The listing builds one solid part. Answer for the finished solid, in the listing's coordinates (mm). Coordinates: 2 decimals unless noted, no trailing zeros. Loops run counter-clockwise (first coordinate to the right, second up) from the corner with the lowest first, then second, coordinate; pieces in that order, holes last. Notation, with made-up numbers: M 10,23 L 15,23 A26 ccw 15,49 Z; hole C 76.5,32 d4. An arc over 180 degrees is marked long. Answer as a JSON object with one key per item and string values. Group by question number.
1. A cutting plane is placed at B-B on x = 2. Give the vertices of the cut face in (y, z).
2. Given pin 1 (6 mm diameter, centred on x = -53.5, y = -24, fed in from +Z); pin 2 (3 mm diameter, centred on x = 16.5, z = 48.5, fed in from +Y); pin 3 (8 mm diameter, centred on y = 22, z = 85.5, fed in from +X); pin 4 (12 mm diameter, centred on x = 22, y = -32.5, fed in from +Z), each flat-ended and moving along its own axis, determine where each tip first touches the part or whether it passes through.
3. A cutting plane is placed at A-A on y = 0. Give the vertices of the cut face in (x, z).
4. A cutting plane is placed at C-C on z = 98.5. Give the vertices of the cut face in (x, y).
5. A cutting plane is placed at D-D on y = 29.5. Give the vertices of the cut face in (x, z).
6. Straight lines are drawn through the part: L1, parallel to Z at x = -23.5, y = -27; L2, parallel to X at y = -11.5, z = 15.5; L3, parallel to Y at x = -52.5, z = 46.5. For each, find the intervals that lie inside material, in ascending order.
from build123d import *

# Parameters (mm, degrees)
F2_T          = -1.2
F3_R          = 17
F4_DEPTH      = 25
F4_DEPTH_BACK = 25


with BuildPart() as f1:
    # F0 (on Front) → F1 (revolve)
    with BuildSketch(Plane.XZ):
        with BuildLine():
            Line((-16.5, 0), (0, 0))
            Line((0, 0), (0, 127))
            Line((0, 127), (-35, 127))
            ThreePointArc((-35, 127), (-68.5223503683, 57.269382033), (-16.5, 0))
        make_face()
    revolve(axis=Axis((0, 0, 63.5), (0, 0, 1)))

    # F2
    f2_openings = [f1.faces().sort_by_distance(p)[0] for p in [
        (0, 0, 127),
    ]]
    offset(amount=F2_T, openings=f2_openings)

    # F3 (on face) → F4 (cut, two sides)
    with BuildSketch(Plane.XY.offset(1.2)) as f4_sk:
        Circle(F3_R)
    extrude(amount=-F4_DEPTH, mode=Mode.SUBTRACT)
    extrude(f4_sk.sketch, amount=F4_DEPTH_BACK, mode=Mode.SUBTRACT)


solid = f1.part
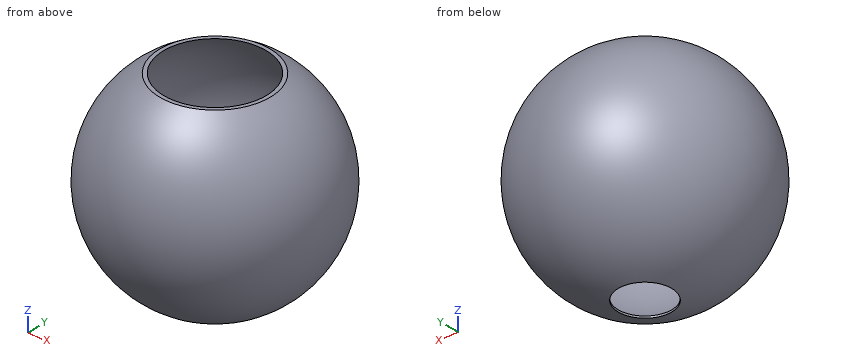
From the geometry:
{
 "1": {"outline": "M -34.94,127 A69.22 ccw -16.88,0.12 L -16.88,1.36 A68.02 cw -32.5,127 Z; M 16.88,0.12 A69.22 ccw 34.94,127 L 32.5,127 A68.02 cw 16.88,1.36 Z"},
 "2": {"pin 1": "stops at z = 108.48", "pin 2": "stops at y = 65.14", "pin 3": "stops at x = 64.73", "pin 4": "stops at z = 127"},
 "3": {"outline": "M -35,127 A69.25 ccw -17,0.12 L -17,1.36 A68.05 cw -32.56,127 Z; M 17,0.12 A69.25 ccw 35,127 L 32.56,127 A68.05 cw 17,1.36 Z"},
 "4": {"outline": "C 0,0 d123.59; hole C 0,0 d120.89"},
 "5": {"outline": "M -18.83,127 A62.65 ccw long 18.83,127 L 13.78,127 A61.32 cw long -13.78,127 Z"},
 "6": {"L1": "z = 7.97 to 9.38, 125.12 to 126.53", "L2": "x = -44.55 to -42.66, 42.66 to 44.55", "L3": "y = -40.1 to -37.99, 37.99 to 40.1"}
}
